Autodesk Inventor part; units mm, degrees
ref_plane "YZ Plane" through (0, 0, 0) normal (1, 0, 0) x (0, 1, 0)
ref_plane "XZ Plane" through (0, 0, 0) normal (0, 1, 0) x (-1, 0, 0)
ref_plane "XY Plane" through (0, 0, 0) normal (0, 0, 1) x (1, 0, 0)
sketch "Block1" plane through (0, 0, 0) normal (0, 0, 1) x (1, 0, 0)
  line L0 (22.5674, 54.9733) -> (22.5674, 26.9733) construction
  line L1 (62.5674, 54.9733) -> (62.5674, 26.9733) construction
  line L2 (42.5674, 54.9733) -> (42.5674, 26.9733) construction
  arc A0 (22.5674, 54.9733) -> (16.0189, 31.9733) centre (39.6923, 37.6653) ccw
  arc A1 (69.116, 31.9733) -> (62.5674, 54.9733) centre (45.4425, 37.6653) ccw
  line L3 (67.5674, 31.9733) -> (69.116, 31.9733)
  line L4 (22.5674, 54.9733) -> (62.5674, 54.9733)
  arc A2 (3.175, 28.049) -> (16.0189, 31.9733) centre (7.7246, 36.1392) ccw
  arc A3 (15.3685, 38.7512) -> (3.175, 28.049) centre (13.5542, 28.5209) ccw
  arc A4 (69.116, 31.9733) -> (81.9598, 28.049) centre (77.4102, 36.1392) ccw
  arc A5 (81.9598, 28.049) -> (69.7664, 38.7512) centre (71.5807, 28.5209) ccw
  line L5 (17.5674, 54.9733) -> (67.5674, 54.9733) construction
  line L6 (67.5674, 54.9733) -> (67.5674, 31.9733) construction
  line L7 (67.5674, 31.9733) -> (16.0189, 31.9733)
  line L8 (17.5674, 31.9733) -> (17.5674, 54.9733) construction
  line L9 (22.5674, 31.9733) -> (62.5674, 31.9733)
  line L10 (62.5674, 31.9733) -> (62.5674, 26.9733)
  line L11 (62.5674, 26.9733) -> (22.5674, 26.9733)
  line L12 (22.5674, 26.9733) -> (22.5674, 31.9733)
  circle A6 centre (35.5674, 51.6287) radius 1
  circle A7 centre (49.5674, 51.6287) radius 1
  line L13 (22.5674, 29.4733) -> (62.5674, 29.4733) construction
  circle A8 centre (35.5674, 29.4733) radius 1
  circle A9 centre (49.5674, 29.4733) radius 1
  point P0 (42.5377, 37.3132)
  point P1 (42.5674, 31.9733)
  point P2 (42.5674, 31.9733)
  point P3 (17.5674, 26.9733)
  point P4 (67.5674, 26.9733)
  dimension "d0" = 23
  dimension "d1" = 5
  dimension "d2" = 40
  dimension "d3" = 2
  dimension "d4" = 2
  dimension "d5" = 7
  dimension "d6" = 7
  dimension "d7" = 2
  dimension "d8" = 2
  dimension "d9" = 7
  dimension "d10" = 7
sketch "Sketch1" plane through (0, 0, 0) normal (0, 0, 1) x (1, 0, 0)
  line L0 (-20, 21.5) -> (-20, -26.5) construction
  line L1 (20, 21.5) -> (20, -26.5) construction
  line L2 (0, 21.5) -> (0, -26.5) construction
  line L3 (27.1698, -21.5) -> (25.1885, -21.5)
  line L4 (-20, 21.5) -> (20, 21.5)
  line L5 (-27.1698, 21.5) -> (27.1698, 21.5) construction
  line L6 (27.1698, 21.5) -> (27.1698, -21.5) construction
  line L7 (27.1698, -21.5) -> (-27.1698, -21.5)
  line L8 (-27.1698, -21.5) -> (-27.1698, 21.5) construction
  line L9 (-20, -21.5) -> (20, -21.5)
  line L10 (20, -21.5) -> (20, -26.5)
  line L11 (20, -26.5) -> (-20, -26.5)
  line L12 (-20, -26.5) -> (-20, -21.5)
  circle A0 centre (-7, 18.1554) radius 1
  circle A1 centre (7, 18.1554) radius 1
  line L13 (-20, -24) -> (20, -24) construction
  circle A2 centre (-7, -24) radius 1
  circle A3 centre (7, -24) radius 1
  circle A4 centre (-17, -18.5) radius 2.25
  circle A5 centre (17, -18.5) radius 2.25
  circle A6 centre (0, -18.5) radius 2.25
  line L14 (-27.1698, 0) -> (27.1698, 0) construction
  circle A7 centre (-7, 0) radius 1
  circle A8 centre (7, 0) radius 1
  circle A9 centre (-7, -18.1554) radius 1
  circle A10 centre (7, -18.1554) radius 1
  arc A11 (-20, 21.5) -> (-27.1698, -21.5) centre (52.9621, -12.7633) ccw
  arc A12 (27.1698, -21.5) -> (20, 21.5) centre (-52.9621, -12.7633) ccw
  arc A13 (-42.2904, -21.5) -> (-27.1698, -21.5) centre (-34.7301, -9.753) ccw
  arc A14 (-27.5757, -9.4306) -> (-42.2904, -21.5) centre (-25.9265, -26.4458) ccw
  arc A15 (27.1698, -21.5) -> (42.2904, -21.5) centre (34.7301, -9.753) ccw
  arc A16 (42.2904, -21.5) -> (27.5757, -9.4306) centre (25.9265, -26.4458) ccw
  point P0 (0, 0)
  point P1 (0, -21.5)
  point P2 (0, -21.5)
  point P3 (-27.9814, 24.963)
  point P4 (27.9814, 24.963)
  point P5 (0, -2.5)
  point P6 (0, 0)
  dimension "d12" = 43
  dimension "d13" = 5
  dimension "d14" = 40
  dimension "d15" = 2
  dimension "d16" = 2
  dimension "d17" = 7
  dimension "d18" = 7
  dimension "d19" = 2
  dimension "d20" = 2
  dimension "d21" = 7
  dimension "d22" = 7
  dimension "d24" = 4.5
  dimension "d25" = 4.5
  dimension "d26" = 3
  dimension "d27" = 3
  dimension "d28" = 3
  dimension "d29" = 3
  dimension "d34" = 4.5
  dimension "d35" = 3
  dimension "d38" = 3.3446
  dimension "d39" = 3.3446
  dimension "d40" = 2
  dimension "d41" = 2
  dimension "d42" = 7
  dimension "d43" = 7
extrude "Extrusion1" add sketch "Sketch1" along normal blind 2 contours L3 L7 A11 L4 A12 | A4 | A5 | A6 | A7 | A8
extrude "Extrusion2" add sketch "Sketch1" along normal blind 0.6 contours A13 A14 A11
mirror "Mirror1" about plane through (0, 0, 0) normal (1, 0, 0) of "Extrusion2"
extrude "Extrusion3" cut sketch "Sketch1" along normal blind 5 contours A4 | A5 | A6
mirror "Mirror2" about plane through (0, 0, 0) normal (0, 1, 0) of "Extrusion3"
extrude "Extrusion4" cut sketch "Sketch1" along normal blind 10 contours A7 | A8
pattern_linear "Rectangular Pattern1" count 3 spacing 6.5 along (0, 1, 0) count 3 spacing 6.5 along (0, -1, 0) of "Extrusion4"
equation "\"d3\" = d11"
equation "\"d4\" = d11"
equation "\"d7\" = d11"
equation "\"d8\" = d11"
equation "\"d15\" = fishing"
equation "\"d16\" = fishing"
equation "\"d19\" = fishing"
equation "\"d20\" = fishing"
equation "\"d40\" = fishing"
equation "\"d41\" = fishing"
equation "\"d11\" = 2"
equation "\"d23\" = 2"
properties part number "Piece"
Input: part model. Units: mm. Frame: model coordinates. A direction names the side the tool comes from. Coordinates: 2 decimals unless noted, no trailing zeros. Loops run counter-clockwise (first coordinate to the right, second up) from the corner with the lowest first, then second, coordinate; pieces in that order, holes last. Notation, with made-up numbers: M 7.25,44.5 L 57.25,44.5 A22 ccw 57.25,53.5 Z; hole C -8.5,40.25 d5. An arc over 180 degrees is marked long. Use a Markdown table: item, result. Add a question column.
1) Line query: L1, parallel to Y at x = 0, z = 1.4; L2, parallel to X at y = 6.5, z = 1.1; L3, parallel to X at y = 0, z = 1. Output: solid intervals per line, ascending. Write a range as from..to.
2) Section C-C, the plane y = 0. Return the cut outline in (x, z).
3) Section B-B, the plane z = 1.3. Give the number of separate pieces and of enclosed holes in the cut face, plus the area to 3 significant figures.
4) Draft query along Y for faces 1 (the flat face through (-1, -6, 0)), 2 (the cylindrical face through (-36.88, -13.32, 0.3)), 3 (the cylindrical face through (-15.962, 20.496, 0.986)). Return one class per face: +Y half, -Y half, draft (parallel to the pull), parting line (faces both ways), or undercut.
5) Pin query (flat end, axial travel): P1, Ø0.6, axis at x = -13.5, z = 1, coming from the -Y side; P2, Ø2, axis at x = 14.5, y = -5.5, coming from the -Z side; P3, Ø1, axis at x = 30.5, z = 0.5, coming from the -Y side. Return the tip coordinate at first contact, or that it passes through.
6) Section A-A, the plane x = 0. Return the cut outline in (y, z), plus the area to 3 significant figures.
7) Set-up query: faces 4 (the cylindrical face through (26.496, 0.799, 0.986)), 5 (the cylindrical face through (-7, -12, 1)). Return all of +Z, -Z, +X, -X, +Y, -Y with unobstructed straight access to the full face (end or side cutting, diameter ignored); none if empty.
8) Section D-D, the plane x = 11.5. Return the cut outline in (y, z), plus the area to 3 significant figures.
Answer below:
| question | item | result |
|---|---|---|
| 1 | L1 | -21.5..-20.75, -16.25..16.25, 20.75..21.5 |
| 1 | L2 | -25.31..-8, -6..6, 8..25.31 |
| 1 | L3 | -26.63..-8, -6..6, 8..26.63 |
| 2 | outline | M -26.63,0 L -8,0 L -8,2 L -26.63,2 Z; M -6,0 L 6,0 L 6,2 L -6,2 Z; M 8,0 L 26.63,0 L 26.63,2 L 8,2 Z |
| 3 | separate pieces | 1 |
| 3 | enclosed holes | 20 |
| 3 | area | 2,060 mm2 |
| 4 | face 1 | draft |
| 4 | face 2 | +Y half |
| 4 | face 3 | undercut |
| 5 | P1 | y = -21.5 |
| 5 | P2 | z = 0 |
| 5 | P3 | y = -23.22 |
| 6 | outline | M -21.5,0 L -20.75,0 L -20.75,2 L -21.5,2 Z; M -16.25,0 L 16.25,0 L 16.25,2 L -16.25,2 Z; M 20.75,0 L 21.5,0 L 21.5,2 L 20.75,2 Z |
| 6 | area | 68.0 mm2 |
| 7 | face 4 | +Z, +X |
| 7 | face 5 | +Z, -Z |
| 8 | outline | M -21.5,0 L 21.5,0 L 21.5,2 L -21.5,2 Z |
| 8 | area | 86.0 mm2 |
